```python
from build123d import *

# Parameters (mm, degrees)
SKETCH_W        = 142
SKETCH_H        = 144
PAD_DEPTH       = 100
SKETCH001_W     = 136
SKETCH001_H     = 30
POCKET_DEPTH    = 95
SKETCH002_W     = 10
SKETCH002_H     = 16
PAD001_DEPTH    = 16
SKETCH003_R     = 4
POCKET001_DEPTH = 4
SKETCH004_R     = 2
POCKET002_DEPTH = 6
SKETCH005_W     = 16
SKETCH005_H     = 10
PAD002_DEPTH    = 16
SKETCH006_R     = 4
POCKET003_DEPTH = 4
SKETCH007_R     = 2
POCKET004_DEPTH = 6
POCKET005_DEPTH = 22
SKETCH009_W     = 10
SKETCH009_H     = 16
PAD003_DEPTH    = 16
SKETCH010_R     = 4
POCKET006_DEPTH = 4
SKETCH011_R     = 2
POCKET007_DEPTH = 6
CHAMFER_SIZE    = 15.98
CHAMFER001_SIZE = 15.98
FILLET_R        = 4
FILLET001_R     = 4
FILLET002_R     = 4
FILLET003_R     = 4
FILLET004_R     = 2
FILLET005_R     = 2
FILLET006_R     = 4


with BuildPart() as part:
    # Sketch → Pad (new body)
    with BuildSketch(Plane.XY):
        with Locations((71, 72)):
            Rectangle(SKETCH_W, SKETCH_H)
    extrude(amount=PAD_DEPTH)

    # Sketch001 (on Face6 of Pad) → Pocket (cut)
    with BuildSketch(Plane.XY.offset(100)):
        with Locations((71, 123)):
            Rectangle(SKETCH001_W, SKETCH001_H)
        with Locations((71, 89)):
            Rectangle(SKETCH001_W, SKETCH001_H)
        with Locations((71, 55)):
            Rectangle(SKETCH001_W, SKETCH001_H)
        with Locations((71, 21)):
            Rectangle(SKETCH001_W, SKETCH001_H)
    extrude(amount=-POCKET_DEPTH, mode=Mode.SUBTRACT)

    # Sketch002 (on Face1 of Pocket) → Pad001 (join)
    with BuildSketch(Plane(origin=(0, 144, 0), x_dir=(-1, 0, 0), z_dir=(0, 1, 0))):
        with Locations((-5, 32)):
            Rectangle(SKETCH002_W, SKETCH002_H)
    extrude(amount=PAD001_DEPTH)

    # Sketch003 (on Face10 of Pad001) → Pocket001 (cut)
    with BuildSketch(Plane(origin=(0, 0, 0), x_dir=(0, -1, 0), z_dir=(-1, 0, 0))):
        with Locations((-152, 32)):
            Circle(SKETCH003_R)
    extrude(amount=-POCKET001_DEPTH, mode=Mode.SUBTRACT)

    # Sketch004 (on Face33 of Pocket001) → Pocket002 (cut)
    with BuildSketch(Plane(origin=(4, 0, 0), x_dir=(0, -1, 0), z_dir=(-1, 0, 0))):
        with Locations((-152, 32)):
            Circle(SKETCH004_R)
    extrude(amount=-POCKET002_DEPTH, mode=Mode.SUBTRACT)

    # Sketch005 (on Face4 of Pocket002) → Pad002 (join)
    with BuildSketch(Plane.XZ):
        with Locations((8, 5)):
            Rectangle(SKETCH005_W, SKETCH005_H)
        with Locations((134, 5)):
            Rectangle(SKETCH005_W, SKETCH005_H)
    extrude(amount=PAD002_DEPTH)

    # Sketch006 (on Face38 of Pad002) → Pocket003 (cut)
    with BuildSketch(Plane.XY.offset(10)):
        with Locations((8, -8)):
            Circle(SKETCH006_R)
        with Locations((134, -8)):
            Circle(SKETCH006_R)
    extrude(amount=-POCKET003_DEPTH, mode=Mode.SUBTRACT)

    # Sketch007 (on Face48 of Pocket003) → Pocket004 (cut)
    with BuildSketch(Plane.XY.offset(6)):
        with Locations((8, -8)):
            Circle(SKETCH007_R)
        with Locations((134, -8)):
            Circle(SKETCH007_R)
    extrude(amount=-POCKET004_DEPTH, mode=Mode.SUBTRACT)

    # Sketch008 (on Face5 of Pocket004) → Pocket005 (cut)
    with BuildSketch(Plane(origin=(0, 0, 0), x_dir=(0, -1, 0), z_dir=(-1, 0, 0))):
        Polygon((-144, 6), (-144, 0), (-138, 0), align=None)
    extrude(amount=-POCKET005_DEPTH, mode=Mode.SUBTRACT)

    # Sketch009 (on Face3 of Pocket005) → Pad003 (join)
    with BuildSketch(Plane.YZ.offset(142)):
        with Locations((5, 92)):
            Rectangle(SKETCH009_W, SKETCH009_H)
    extrude(amount=PAD003_DEPTH)

    # Sketch010 (on Face42 of Pad003) → Pocket006 (cut)
    with BuildSketch(Plane.XZ):
        with Locations((150, 92)):
            Circle(SKETCH010_R)
    extrude(amount=-POCKET006_DEPTH, mode=Mode.SUBTRACT)

    # Sketch011 (on Face59 of Pocket006) → Pocket007 (cut)
    with BuildSketch(Plane.XZ.offset(-4)):
        with Locations((150, 92)):
            Circle(SKETCH011_R)
    extrude(amount=-POCKET007_DEPTH, mode=Mode.SUBTRACT)

    # Chamfer
    chamfer_edges = [part.edges().sort_by_distance(p)[0] for p in [
        (5, 144, 24),
    ]]
    chamfer(chamfer_edges, length=CHAMFER_SIZE)

    # Chamfer001
    chamfer001_edges = [part.edges().sort_by_distance(p)[0] for p in [
        (142, 5, 84),
    ]]
    chamfer(chamfer001_edges, length=CHAMFER001_SIZE)

    # Fillet
    fillet_edges = [part.edges().sort_by_distance(p)[0] for p in [
        (0, 0, 55),
    ]]
    fillet(fillet_edges, radius=FILLET_R)

    # Fillet001
    fillet001_edges = [part.edges().sort_by_distance(p)[0] for p in [
        (142, -16, 5),
        (126, -16, 5),
        (16, -16, 5),
        (0, -16, 5),
    ]]
    fillet(fillet001_edges, radius=FILLET001_R)

    # Fillet002
    fillet002_edges = [part.edges().sort_by_distance(p)[0] for p in [
        (142, 0, 39.01),
    ]]
    fillet(fillet002_edges, radius=FILLET002_R)

    # Fillet003
    fillet003_edges = [part.edges().sort_by_distance(p)[0] for p in [
        (158, 5, 100),
    ]]
    fillet(fillet003_edges, radius=FILLET003_R)

    # Fillet004
    fillet004_edges = [part.edges().sort_by_distance(p)[0] for p in [
        (0, 144, 70),
    ]]
    fillet(fillet004_edges, radius=FILLET004_R)

    # Fillet005
    fillet005_edges = [part.edges().sort_by_distance(p)[0] for p in [
        (142, 144, 50),
    ]]
    fillet(fillet005_edges, radius=FILLET005_R)

    # Fillet006
    fillet006_edges = [part.edges().sort_by_distance(p)[0] for p in [
        (5, 160, 40),
    ]]
    fillet(fillet006_edges, radius=FILLET006_R)


solid = part.part
```
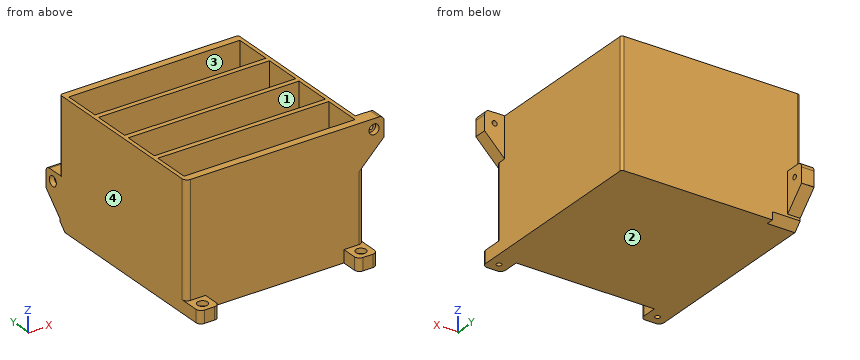
Geometry: final body of the model. Coordinates: model frame, mm. Face numbers are marked on the shaded views. A direction names the side the tool comes from. Coordinates: 2 decimals unless noted, no trailing zeros. Order: outer loops, then holes, each group sorted by start corner. A loop starts at its lowest first (then second) coordinate and runs counter-clockwise, first axis right, second up. Notation, with made-up numbers: (37, 33) - (65, 33) arc R18 cw to (65, 66) - close; hole circle Ø5 at (42, 29). An arc over 180 degrees is marked (long way). Write each question's results on one line, items separated by ' | '.
(1) Section query D-D, the plane z = 78.5. Return the cut outline in (x, y).
Values found:
outline: (0, 4) arc R4 ccw to (4, 0) - (152.48, 0) - (152.48, 10) - (142, 10) - (142, 142) arc R2 ccw to (140, 144) - (2, 144) arc R2 ccw to (0, 142) - close; hole (3, 6) - (139, 6) - (139, 36) - (3, 36) - close; hole (3, 40) - (139, 40) - (139, 70) - (3, 70) - close; hole (3, 74) - (139, 74) - (139, 104) - (3, 104) - close; hole (3, 108) - (139, 108) - (139, 138) - (3, 138) - close
(2) Section query B-B, the plane y = 60. Return the cut outline in (x, z), plus the area to 3 significant figures.
Values found:
outline: (0, 0) - (142, 0) - (142, 100) - (139, 100) - (139, 5) - (3, 5) - (3, 100) - (0, 100) - close | area: 1,280 mm²
(3) Set-up query: the marked faces 1 and 2. Return all of +Z, -Z, +X, -X, +Y, -Y with unobstructed straight access to the full face (end or side cutting, diameter ignored); none if empty.
Values found:
face 1: +Z | face 2: -Z, +X, -X, +Y, -Y
(4) Section query A-A, the plane z = 44. Return the cut outline in (x, y).
Values found:
outline: (0, 4) arc R4 ccw to (4, 0) - (138, 0) arc R4 ccw to (142, 4) - (142, 142) arc R2 ccw to (140, 144) - (2, 144) arc R2 ccw to (0, 142) - close; hole (3, 6) - (139, 6) - (139, 36) - (3, 36) - close; hole (3, 40) - (139, 40) - (139, 70) - (3, 70) - close; hole (3, 74) - (139, 74) - (139, 104) - (3, 104) - close; hole (3, 108) - (139, 108) - (139, 138) - (3, 138) - close
(5) First-contact query: pin 1 Ø8 at (x, y) = (11.5, -10) entering from +Z; pin 2 Ø8 at (x, y) = (5, 149) entering from +Z; pin 3 Ø9 at (x, y) = (83.5, 22.5) entering from +Z. Flat tips, straight axial feed; report the tip coordinate or a pass-through.
Values found:
pin 1: stops at z = 10 | pin 2: stops at z = 40 | pin 3: stops at z = 5
(6) Section query C-C, the plane x = 82.5. Return the cut outline in (y, z).
Values found:
outline: (0, 0) - (144, 0) - (144, 100) - (138, 100) - (138, 5) - (108, 5) - (108, 100) - (104, 100) - (104, 5) - (74, 5) - (74, 100) - (70, 100) - (70, 5) - (40, 5) - (40, 100) - (36, 100) - (36, 5) - (6, 5) - (6, 100) - (0, 100) - close
(7) Line query: line 1 (Y direction, x = 59.5, z = 76); line 2 (Y direction, x = 8, z = 7.3); line 3 (X direction, y = 27, z = 32.5). Output: solid intervals per line, ascending. Write a range as [from, to].
Values found:
line 1: y = [0, 6], [36, 40], [70, 74], [104, 108], [138, 144] | line 2: y = [-16, -12], [-4, 6], [36, 40], [70, 74], [104, 108], [138, 144] | line 3: x = [0, 3], [139, 142]
(8) Mould query, pull axis Y, two halves, no side actions, for the marked faces 3 and 4. Classes: +Y half, -Y half, draft (parallel to the pull), parting line (faces both ways), or undercut.
Values found:
face 3: undercut | face 4: draft
